```python
from build123d import *

# Parameters (mm, degrees)
SKETCH_R   = 2
SKETCH_R_2 = 1.5
PAD_DEPTH  = 3


with BuildPart() as part:
    # Sketch → Pad (new body)
    with BuildSketch(Plane.XY):
        Polygon((87, 0), (87, 91.15), (17, 91.15), (17, 30.85), (0, 30.85), (0, 11.5), (11.5, 11.5), (11.5, 0), align=None)
        with Locations((27, 71.15)):
            Circle(SKETCH_R, mode=Mode.SUBTRACT)
        with Locations((58, 71.15)):
            Circle(SKETCH_R, mode=Mode.SUBTRACT)
        with Locations((58, 46.85)):
            Circle(SKETCH_R, mode=Mode.SUBTRACT)
        with Locations((27, 46.85)):
            Circle(SKETCH_R, mode=Mode.SUBTRACT)
        with Locations((21.7, 5)):
            Circle(SKETCH_R_2, mode=Mode.SUBTRACT)
        with Locations((29.7, 5)):
            Circle(SKETCH_R_2, mode=Mode.SUBTRACT)
        with Locations((70.3, 8.7)):
            Circle(SKETCH_R_2, mode=Mode.SUBTRACT)
        with Locations((62.3, 8.7)):
            Circle(SKETCH_R_2, mode=Mode.SUBTRACT)
        with Locations((22.7, 85.45)):
            Circle(SKETCH_R_2, mode=Mode.SUBTRACT)
        with Locations((67, 85.45)):
            Circle(SKETCH_R_2, mode=Mode.SUBTRACT)
        with Locations((27.5, 22)):
            Circle(SKETCH_R_2, mode=Mode.SUBTRACT)
        with Locations((44.5, 22)):
            Circle(SKETCH_R_2, mode=Mode.SUBTRACT)
        with Locations((61.5, 22)):
            Circle(SKETCH_R_2, mode=Mode.SUBTRACT)
        with Locations((78.5, 22)):
            Circle(SKETCH_R_2, mode=Mode.SUBTRACT)
        with Locations((12, 22.85)):
            Circle(SKETCH_R_2, mode=Mode.SUBTRACT)
        with Locations((40, 12)):
            Circle(SKETCH_R_2, mode=Mode.SUBTRACT)
        Polygon((68, 59), (68, 66.5), (53, 66.5), (53, 51.5), (68, 51.5), align=None, mode=Mode.SUBTRACT)
    pad = extrude(amount=PAD_DEPTH)

    # Mirrored: Pad across face of Pad
    add(pad.mirror(Plane(origin=(87, 45.575, 1.5), x_dir=(0, 1, 0), z_dir=(1, 0, 0))))


solid = part.part
```
Work out the finished part from the listing and answer in its coordinate system (mm). A direction names the side the tool comes from. Round coordinates to 2 decimals unless told otherwise and drop trailing zeros. Loops run counter-clockwise (first coordinate to the right, second up) from the corner with the lowest first, then second, coordinate; pieces in that order, holes last.
(1) Find the intervals of material crossed by L1, parallel to X at y = 9, z = 1.6; L2, parallel to Y at x = 58, z = 0.8; L3, parallel to X at y = 46.5, z = 2.8, in increasing order.
Computed values:
L1: x = 11.5 to 60.83, 63.77 to 68.83, 71.77 to 102.23, 105.17 to 110.23, 113.17 to 162.5
L2: y = 0 to 44.85, 48.85 to 51.5, 66.5 to 69.15, 73.15 to 91.15
L3: x = 17 to 25.03, 28.97 to 56.03, 59.97 to 114.03, 117.97 to 145.03, 148.97 to 157
(2) Each of these flat-tipped pins is pushed along its axis until it touches: P1, Ø1.5, axis at x = 164.5, z = 2, coming from the +Y side; P2, Ø1.5, axis at y = 4, z = 1.5, coming from the +X side; P3, Ø1, axis at y = 75.5, z = 1.5, coming from the +X side. Where does it stop, or does it pass through?
Computed values:
P1: stops at y = 30.85
P2: stops at x = 162.5
P3: stops at x = 157
(3) The part is cut by section B-B, the plane z = 2.35. Give the number of separate pieces and of enclosed holes in the cut face, and give its area (3 significant figures).
Computed values:
separate pieces: 1
enclosed holes: 34
area: 12,800 mm2
(4) For faces 3 (the flat face through (88, 46, 0)), 4 (the flat face through (53, 59, 1)), determine the directions among +Z, -Z, +X, -X, +Y, -Y from which every point of the face is accessible in a straight line to the end or side of a thin tool.
Computed values:
face 3: -Z, +X, -X, +Y, -Y
face 4: +Z, -Z
(5) The mould has two halves that part along Y. Classify faces 1 (the flat face through (174, 21, 1)), 2 (the cylindrical face through (117.587, 69.933, 1.479)): pulls with the +Y half, pulls with the -Y half, needs draft (parallel to the pull), parting line crosses it, or undercut.
Computed values:
face 1: needs draft
face 2: undercut
(6) The part is cut by section A-A, the plane y = 46.85. Give the vertices of the cut face in (x, z).
Computed values:
outline: (17, 0) - (25, 0) - (25, 3) - (17, 3) - close; (29, 0) - (56, 0) - (56, 3) - (29, 3) - close; (60, 0) - (114, 0) - (114, 3) - (60, 3) - close; (118, 0) - (145, 0) - (145, 3) - (118, 3) - close; (149, 0) - (157, 0) - (157, 3) - (149, 3) - close
